Could you check a few things on this drawing? It's one solid part, dimensions in mm from its lowest x, y, z. Give positions to 0.01 mm unless a question says otherwise; leave off trailing zeros. Order: outer loops, then holes, each group sorted by start corner. A loop starts at its lowest first (then second) coordinate and runs counter-clockwise, first axis right, second up.
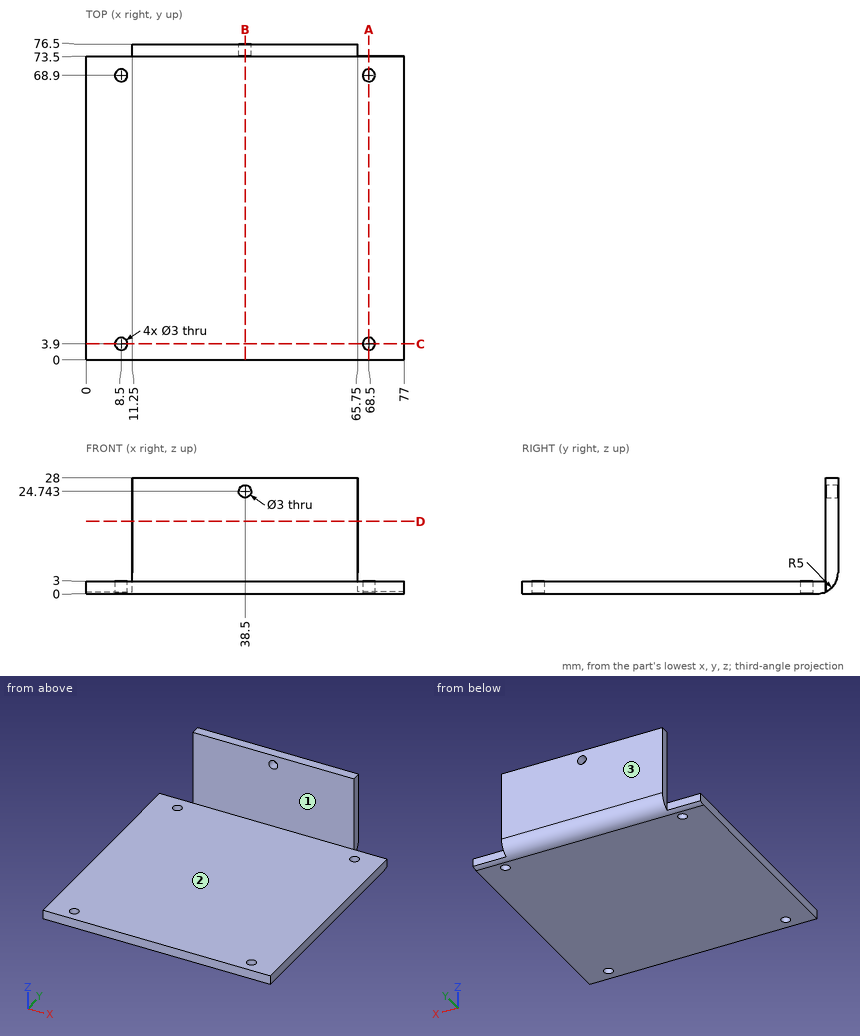
Item 1: Please list where these lines run through material, in increasing order: line 1 along X through (y, z) = (68.9, 1.3); line 2 along Y through (x, z) = (8.5, 0.7); line 3 along Z through (x, y) = (23.5, 60.5).
Findings:
line 1: x = 0 to 7, 10 to 67, 70 to 77
line 2: y = 0 to 2.4, 5.4 to 67.4, 70.4 to 73.5
line 3: z = 0 to 3
Item 2: We'd pull the mould along Y, two halves only. Please class the marked faces 1, 2 and 3: +Y half, -Y half, draft (parallel to the pull), parting line (faces both ways), or undercut.
Findings:
face 1: -Y half
face 2: draft
face 3: +Y half
Item 3: Imagine slicing it at A-A on x = 68.5. List the corners of the cut face in (y, z) for me, then the cut area to 3 significant figures.
Findings:
outline: (0, 0) - (2.4, 0) - (2.4, 3) - (0, 3) - close; (5.4, 0) - (67.4, 0) - (67.4, 3) - (5.4, 3) - close; (70.4, 0) - (71.5, 0) arc R5 ccw to (73.5, 0.42) - (73.5, 3) - (70.4, 3) - close
area: 202 mm2
Item 4: Imagine slicing it at B-B on x = 38.5. List the corners of the cut face in (y, z) for me, then the cut area to 3 significant figures.
Findings:
outline: (0, 0) - (71.5, 0) arc R5 ccw to (76.5, 5) - (76.5, 23.24) - (73.5, 23.24) - (73.5, 3) - (0, 3) - close; (73.5, 26.24) - (76.5, 26.24) - (76.5, 28) - (73.5, 28) - close
area: 290 mm2
Item 5: For pin 1 (0.8 mm diameter, centred on x = 4, z = 2, fed in from +Y); pin 2 (2.5 mm diameter, centred on x = 68.5, y = 3.9, fed in from -Z); pin 3 (0.9 mm diameter, centred on y = 75, z = 7.5, fed in from -X); pin 4 (1.5 mm diameter, centred on y = 74.5, z = 13.5, fed in from +X), each with a flat end and sliding along its axis, tell me the tip position at first contact or that it passes through.
Findings:
pin 1: stops at y = 73.5
pin 2: passes through
pin 3: stops at x = 11.25
pin 4: stops at x = 65.75
Item 6: Imagine slicing it at C-C on y = 3.9. List the corners of the cut face in (x, z) for me.
Findings:
outline: (0, 0) - (7, 0) - (7, 3) - (0, 3) - close; (10, 0) - (67, 0) - (67, 3) - (10, 3) - close; (70, 0) - (77, 0) - (77, 3) - (70, 3) - close
Item 7: Imagine slicing it at D-D on z = 17.5. List the corners of the cut face in (x, y) for me.
Findings:
outline: (11.25, 73.5) - (65.75, 73.5) - (65.75, 76.5) - (11.25, 76.5) - close
